The model under review builds one solid part; all positions refer to its coordinate system, in mm. A direction names the side the tool comes from. Coordinates: 2 decimals unless noted, no trailing zeros. Loops run counter-clockwise (first coordinate to the right, second up) from the corner with the lowest first, then second, coordinate; pieces in that order, holes last. Notation, with made-up numbers: (59, 43) - (118, 43) arc R15 ccw to (118, 69) - close; hole circle Ø4 at (86.25, 58.25). An arc over 180 degrees is marked (long way). One line per item, written item: value. Start each with the question number.
1. We need section A-A, the plane x = 24. Give the boundary of the cut face in (y, z).
2. Insertion check: P1, Ø6, axis at x = 55, z = 55.5, coming from the -Y side; P2, Ø4, axis at y = 8.5, z = 11.5, coming from the +X side. Each pin has a flat end and moves straight along its axis. Give the tip position at first contact, or say it passes through.
3. We need section B-B, the plane z = 46. Give the boundary of the cut face in (x, y), then the cut area to 3 significant figures.
4. Mouldability with a two-part tool opening along X and no side actions: class faces 1 (the face through (0, 20, 51)), 2 (the face through (49, 40, 49)), 3 (the face through (99, 19, 49)) as +X half, -X half, draft (parallel to the pull), parting line (faces both ways), or undercut.
5. We need section D-D, the plane z = 32.5. Give the boundary of the cut face in (x, y), then the cut area to 4 significant figures.
6. To check wall thickness, follow line 1 (Z direction, x = 27.5, y = 31); line 2 (Y direction, x = 14.5, z = 37). State the ranges of each line that lie inside material, in increasing order.
7. For faces 4 (the face through (51, 20, 100)), 5 (the face through (49, 39, 49)), list the 3-axis set-ups (+Z, -Z, +X, -X, +Y, -Y) from which the entire face can be reached by the end or side of a thin tool; tool diameter is ignored.
8. We need section C-C, the plane y = 33. Give the boundary of the cut face in (x, z).
Autodesk Fusion 360 part; units mm, degrees
sketch "Sketch1" plane through (0, 0, 0) normal (0, 1, 0) x (1, 0, 0) in component "Outer Hull"
  line L0 (0, 0) -> (100, 0)
  line L1 (100, 0) -> (100, -100)
  line L2 (100, -100) -> (0, -100)
  line L3 (0, -100) -> (0, 0)
  dimension "d1" = 100
  dimension "d2" = 100
extrude "Extrude1" add sketch "Sketch1" along normal blind 40 in component "Outer Hull"
shell "Shell1" thickness 1 removed faces 1 at (33.3333, 0, 33.3333) in component "Outer Hull"
sketch "Button hole" plane through (0, 40, 0) normal (0, 1, 0) x (-1, 0, 0)
  line L0 (0, 100) -> (-100, 100)
  line L1 (-100, 100) -> (-100, 0)
  line L2 (-100, 0) -> (0, 0)
  line L3 (0, 0) -> (0, 100)
  line L4 (-7, 5) -> (-13, 5)
  line L5 (-15, 7) -> (-15, 18)
  line L6 (-13, 20) -> (-7, 20)
  line L7 (-5, 18) -> (-5, 7)
  arc A0 (-7, 5) -> (-5, 7) centre (-7, 7) ccw
  arc A1 (-15, 7) -> (-13, 5) centre (-13, 7) ccw
  arc A2 (-13, 20) -> (-15, 18) centre (-13, 18) ccw
  arc A3 (-5, 18) -> (-7, 20) centre (-7, 18) ccw
  dimension "d6" = 2
extrude "Extrude2" cut sketch "Button hole" against normal blind 1 contours L4 L5 L6 L7 A0 A1 A2 A3 in component "Outer Hull"
pattern_linear "R-Pattern1" count 3 spacing 17.5 along (0, 0, 1) count 2 spacing 15 along (1, 0, 0) of "Extrude2" in component "Outer Hull"
sketch "Top toggle" plane through (0, 40, 0) normal (0, 1, 0) x (-1, 0, 0)
  line L0 (-20, 18) -> (-20, 7)
  arc A0 (-22, 5) -> (-20, 7) centre (-22, 7) ccw
  line L1 (-22, 5) -> (-28, 5)
  arc A1 (-30, 7) -> (-28, 5) centre (-28, 7) ccw
  line L2 (-30, 7) -> (-30, 18)
  arc A2 (-28, 20) -> (-30, 18) centre (-28, 18) ccw
  line L3 (-28, 20) -> (-22, 20)
  arc A3 (-20, 18) -> (-22, 20) centre (-22, 18) ccw
  line L4 (-5, 18) -> (-5, 7)
  arc A4 (-7, 5) -> (-5, 7) centre (-7, 7) ccw
  line L5 (-7, 5) -> (-13, 5)
  arc A5 (-15, 7) -> (-13, 5) centre (-13, 7) ccw
  line L6 (-15, 7) -> (-15, 18)
  arc A6 (-13, 20) -> (-15, 18) centre (-13, 18) ccw
  line L7 (-13, 20) -> (-7, 20)
  arc A7 (-5, 18) -> (-7, 20) centre (-7, 18) ccw
  line L8 (0, 100) -> (-100, 100)
  line L9 (-100, 100) -> (-100, 0)
  line L10 (-100, 0) -> (0, 0)
  line L11 (0, 0) -> (0, 100)
  line L12 (-45, 10) -> (-55, 10)
  line L13 (-55, 10) -> (-55, 12.5)
  line L14 (-55, 12.5) -> (-45, 12.5)
  line L15 (-45, 12.5) -> (-45, 10)
  line L16 (-20, 53) -> (-20, 42)
  arc A8 (-22, 40) -> (-20, 42) centre (-22, 42) ccw
  line L17 (-22, 40) -> (-28, 40)
  arc A9 (-30, 42) -> (-28, 40) centre (-28, 42) ccw
  line L18 (-30, 42) -> (-30, 53)
  arc A10 (-28, 55) -> (-30, 53) centre (-28, 53) ccw
  line L19 (-28, 55) -> (-22, 55)
  arc A11 (-20, 53) -> (-22, 55) centre (-22, 53) ccw
  line L20 (-20, 35.5) -> (-20, 24.5)
  arc A12 (-22, 22.5) -> (-20, 24.5) centre (-22, 24.5) ccw
  line L21 (-22, 22.5) -> (-28, 22.5)
  arc A13 (-30, 24.5) -> (-28, 22.5) centre (-28, 24.5) ccw
  line L22 (-30, 24.5) -> (-30, 35.5)
  arc A14 (-28, 37.5) -> (-30, 35.5) centre (-28, 35.5) ccw
  line L23 (-28, 37.5) -> (-22, 37.5)
  arc A15 (-20, 35.5) -> (-22, 37.5) centre (-22, 35.5) ccw
  line L24 (-5, 53) -> (-5, 42)
  arc A16 (-7, 40) -> (-5, 42) centre (-7, 42) ccw
  line L25 (-7, 40) -> (-13, 40)
  arc A17 (-15, 42) -> (-13, 40) centre (-13, 42) ccw
  line L26 (-15, 42) -> (-15, 53)
  arc A18 (-13, 55) -> (-15, 53) centre (-13, 53) ccw
  line L27 (-13, 55) -> (-7, 55)
  arc A19 (-5, 53) -> (-7, 55) centre (-7, 53) ccw
  line L28 (-5, 35.5) -> (-5, 24.5)
  arc A20 (-7, 22.5) -> (-5, 24.5) centre (-7, 24.5) ccw
  line L29 (-7, 22.5) -> (-13, 22.5)
  arc A21 (-15, 24.5) -> (-13, 22.5) centre (-13, 24.5) ccw
  line L30 (-15, 24.5) -> (-15, 35.5)
  arc A22 (-13, 37.5) -> (-15, 35.5) centre (-13, 35.5) ccw
  line L31 (-13, 37.5) -> (-7, 37.5)
  arc A23 (-5, 35.5) -> (-7, 37.5) centre (-7, 35.5) ccw
  dimension "d17" = 10
  dimension "d18" = 2.5
extrude "Extrude3" cut sketch "Top toggle" against normal blind 1 contours L12 L13 L14 L15 in component "Outer Hull"
sketch "Wire inlet" plane through (100, 0, 0) normal (1, 0, 0) x (0, 0, -1)
  line L0 (-100, 0) -> (0, 0)
  line L1 (0, 0) -> (0, 40)
  line L2 (0, 40) -> (-100, 40)
  line L3 (-100, 40) -> (-100, 0)
  line L4 (-7, 5) -> (-18, 5)
  line L5 (-20, 7) -> (-20, 18)
  line L6 (-18, 20) -> (-7, 20)
  line L7 (-5, 18) -> (-5, 7)
  arc A0 (-18, 20) -> (-20, 18) centre (-18, 18) ccw
  arc A1 (-5, 18) -> (-7, 20) centre (-7, 18) ccw
  arc A2 (-7, 5) -> (-5, 7) centre (-7, 7) ccw
  arc A3 (-20, 7) -> (-18, 5) centre (-18, 7) ccw
  dimension "d21" = 2
extrude "Extrude4" cut sketch "Wire inlet" against normal blind 1 contours L4 L5 L6 L7 A0 A1 A2 A3 in component "Outer Hull"
sketch "Sketch4" plane through (100, 0, 0) normal (1, 0, 0) x (0, 0, -1)
  line L0 (-20, 7) -> (-20, 18)
  arc A0 (-18, 20) -> (-20, 18) centre (-18, 18) ccw
  line L1 (-18, 20) -> (-7, 20)
  arc A1 (-5, 18) -> (-7, 20) centre (-7, 18) ccw
  line L2 (-5, 18) -> (-5, 7)
  arc A2 (-7, 5) -> (-5, 7) centre (-7, 7) ccw
  line L3 (-7, 5) -> (-18, 5)
  arc A3 (-20, 7) -> (-18, 5) centre (-18, 7) ccw
  line L4 (-100, 0) -> (0, 0)
  line L5 (0, 0) -> (0, 40)
  line L6 (0, 40) -> (-100, 40)
  line L7 (-100, 40) -> (-100, 0)
  line L8 (-25, 5) -> (-35, 5)
  line L9 (-35, 5) -> (-35, 7.5)
  line L10 (-35, 7.5) -> (-25, 7.5)
  line L11 (-25, 7.5) -> (-25, 5)
  dimension "d24" = 10
  dimension "d25" = 2.5
extrude "Extrude5" cut sketch "Sketch4" against normal blind 1 contours L8 L9 L10 L11 in component "Outer Hull"
component "Outer Hull" placed x (1, 0, 0) y (0, 1, 0) z (0, 0, 1) at (0, 0, 0)
Findings below:
1. outline: (0, 0) - (40, 0) - (40, 5) - (39, 5) - (39, 1) - (0, 1) - close; (0, 99) - (39, 99) - (39, 55) - (40, 55) - (40, 100) - (0, 100) - close; (39, 20) - (40, 20) - (40, 22.5) - (39, 22.5) - close; (39, 37.5) - (40, 37.5) - (40, 40) - (39, 40) - close
2. P1: y = 39
2. P2: x = 1
3. outline: (0, 0) - (1, 0) - (1, 39) - (5, 39) - (5, 40) - (0, 40) - close; (15, 39) - (20, 39) - (20, 40) - (15, 40) - close; (30, 39) - (99, 39) - (99, 0) - (100, 0) - (100, 40) - (30, 40) - close
3. area: 158 mm2
4. face 1: -X half
4. face 2: draft
4. face 3: undercut
5. outline: (0, 0) - (1, 0) - (1, 39) - (5, 39) - (5, 40) - (0, 40) - close; (15, 39) - (20, 39) - (20, 40) - (15, 40) - close; (30, 39) - (99, 39) - (99, 7.5) - (100, 7.5) - (100, 40) - (30, 40) - close; (99, 0) - (100, 0) - (100, 5) - (99, 5) - close
5. area: 155.5 mm2
6. line 1: 0 to 1, 99 to 100
6. line 2: 39 to 40
7. face 4: +Z, +X, -X, +Y, -Y
7. face 5: -Y
8. outline: (0, 0) - (100, 0) - (100, 100) - (0, 100) - close; hole (1, 1) - (99, 1) - (99, 99) - (1, 99) - close
